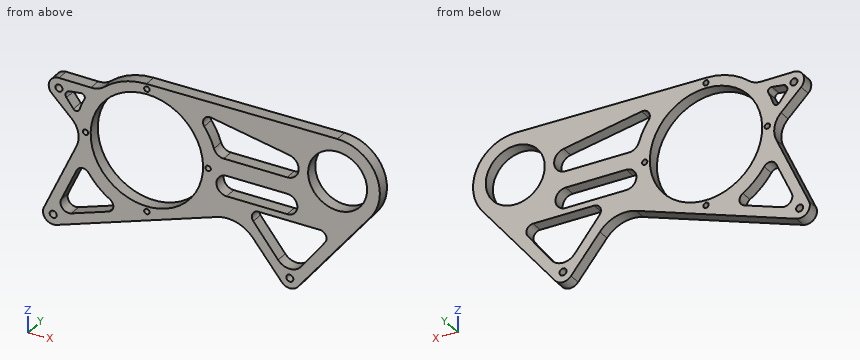
from build123d import *

# Parameters (mm, degrees)
SKETCH1_R             = 52.3875
SKETCH1_R_2           = 27.49999999
BOSS_EXTRUDE1_DEPTH   = 11.43
M6_CLEARANCE_HOLE1_D  = 6.6
F_5_0MM_DOWEL_HOLE1_D = 5
CIRPATTERN1_COUNT     = 4
CUT_EXTRUDE1_DEPTH    = 277.04812471
CUT_EXTRUDE2_DEPTH    = 277.04812471


with BuildPart() as part:
    # Sketch1 → Boss-Extrude1 (new body)
    with BuildSketch(Plane(origin=(0, 0, 0), x_dir=(1, 0, 0), z_dir=(0, 1, 0))):
        with BuildLine():
            Line((-207.352675902, -8.773903901), (-58.019530206, -60.290898352))
            ThreePointArc((-58.019530206, -60.290898352), (-39.599212065, -60.776397748), (-24.240097525, -50.595954211))
            Line((-24.240097525, -50.595954211), (2.624995443, -17.347825368))
            ThreePointArc((2.624995443, -17.347825368), (10.061549983, -13.809238065), (17.477288292, -17.391244328))
            Line((17.477288292, -17.391244328), (85.376811489, -102.435794114))
            ThreePointArc((85.376811489, -102.435794114), (90.030312626, -144.187156643), (54.354134393, -166.369168556))
            Line((54.354134393, -166.369168556), (-123.592369302, -165.212669907))
            ThreePointArc((-123.592369302, -165.212669907), (-144.74612022, -161.34018293), (-163.299086644, -150.465222234))
            ThreePointArc((-163.299086644, -150.465222234), (-168.867064733, -147.400846083), (-175.155117318, -146.477170878))
            Line((-175.155117318, -146.477170878), (-205.054266123, -146.707116576))
            ThreePointArc((-205.054266123, -146.707116576), (-213.929698734, -140.822073907), (-211.802405396, -130.387436669))
            Line((-211.802405396, -130.387436669), (-193.092894011, -112.008542149))
            ThreePointArc((-193.092894011, -112.008542149), (-187.088381157, -100.6982482), (-188.678110669, -87.991962988))
            Line((-188.678110669, -87.991962988), (-219.113977597, -21.755141651))
            ThreePointArc((-219.113977597, -21.755141651), (-217.51766362, -11.382814462), (-207.352675902, -8.773903901))
        make_face()
        with Locations(Location((-123.19, -103.30147742, 0), (0, 0, 270))):
            Circle(SKETCH1_R, mode=Mode.SUBTRACT)
        with Locations(Location((54.61, -127, 0), (0, 0, 270))):
            Circle(SKETCH1_R_2, mode=Mode.SUBTRACT)
    extrude(amount=BOSS_EXTRUDE1_DEPTH)

    # M6 Clearance Hole1 (through all)
    with Locations(Plane(origin=(0, 0, 0), x_dir=(-1, 0, 0), z_dir=(0, -1, 0))):
        with Locations((-10.033704867, -23.334197365), (210.458966133, -17.778157673), (205.127517975, -137.182398252)):
            Hole(M6_CLEARANCE_HOLE1_D / 2)

    # Ø5.0mm Dowel Hole1 (through all)
    with Locations(Plane(origin=(0, 0, 0), x_dir=(-1, 0, 0), z_dir=(0, -1, 0))):
        with Locations((123.19, -160.45147742)):
            f_5_0mm_dowel_hole1 = Hole(F_5_0MM_DOWEL_HOLE1_D / 2)

    # CirPattern1: Ø5.0mm Dowel Hole1 ×4 about axis
    cirpattern1_axis = Axis((-123.19, 0, 103.30147742), (0, 1, 0))
    for i in range(1, CIRPATTERN1_COUNT):
        add(f_5_0mm_dowel_hole1.rotate(cirpattern1_axis, i * 360 / CIRPATTERN1_COUNT), mode=Mode.SUBTRACT)

    # Sketch6 → Cut-Extrude1 (cut, through all)
    with BuildSketch(Plane.XZ):
        with BuildLine():
            Line((-23.944258321, 66.390441023), (-0.829614149, 37.099993387))
            ThreePointArc((-0.829614149, 37.099993387), (9.965816041, 31.919797806), (20.677978855, 37.270060145))
            Line((20.677978855, 37.270060145), (42.980839674, 66.469760223))
            ThreePointArc((42.980839674, 66.469760223), (43.626492897, 73.139052969), (37.934473227, 76.674197365))
            Line((37.934473227, 76.674197365), (-18.959475373, 76.674197365))
            ThreePointArc((-18.959475373, 76.674197365), (-24.673574285, 73.093957935), (-23.944258321, 66.390441023))
        make_face()
        with BuildLine():
            Line((-202.975515938, 34.064204485), (-188.656140545, 65.227105539))
            ThreePointArc((-188.656140545, 65.227105539), (-183.31891043, 68.976517371), (-177.425759363, 66.18100581))
            ThreePointArc((-177.425759363, 66.18100581), (-168.46871459, 55.664464381), (-157.511328264, 47.252450377))
            ThreePointArc((-157.511328264, 47.252450377), (-154.454895213, 41.026593051), (-158.781442678, 35.605885581))
            Line((-158.781442678, 35.605885581), (-193.515753631, 23.623232324))
            ThreePointArc((-193.515753631, 23.623232324), (-201.691580607, 25.721611775), (-202.975515938, 34.064204485))
        make_face()
        with BuildLine():
            Line((-195.382759208, 137.08408238), (-184.602414462, 138.548107412))
            ThreePointArc((-184.602414462, 138.548107412), (-181.561941078, 137.21737146), (-181.352428173, 133.905054912))
            ThreePointArc((-181.352428173, 133.905054912), (-183.92504724, 128.415239444), (-185.980839898, 122.711717787))
            ThreePointArc((-185.980839898, 122.711717787), (-188.468463156, 120.514659048), (-191.560851772, 121.719843357))
            Line((-191.560851772, 121.719843357), (-198.159072812, 130.369853834))
            ThreePointArc((-198.159072812, 130.369853834), (-198.701393345, 134.525214763), (-195.382759208, 137.08408238))
        make_face()
    extrude(amount=-CUT_EXTRUDE1_DEPTH, mode=Mode.SUBTRACT)

    # Sketch7 → Cut-Extrude2 (cut, through all)
    with BuildSketch(Plane.XZ):
        with BuildLine():
            Line((-48.815667356, 101.39647742), (7.572332644, 101.39647742))
            ThreePointArc((7.572332644, 101.39647742), (17.097332644, 91.87147742), (7.572332644, 82.34647742))
            Line((7.572332644, 82.34647742), (-48.815667356, 82.34647742))
            ThreePointArc((-48.815667356, 82.34647742), (-58.340667356, 91.87147742), (-48.815667356, 101.39647742))
        make_face()
        with BuildLine():
            Line((-63.185512617, 151.524232803), (9.527948512, 138.12987842))
            ThreePointArc((9.527948512, 138.12987842), (18.322585695, 126.531617281), (7.572332644, 116.718495252))
            Line((7.572332644, 116.718495252), (-51.525154545, 116.718495252))
            ThreePointArc((-51.525154545, 116.718495252), (-57.140513894, 118.54977285), (-60.59665397, 123.339442362))
            ThreePointArc((-60.59665397, 123.339442362), (-64.418746701, 132.718934684), (-69.636607751, 141.399786896))
            ThreePointArc((-69.636607751, 141.399786896), (-69.82125671, 148.634919104), (-63.185512617, 151.524232803))
        make_face()
    extrude(amount=-CUT_EXTRUDE2_DEPTH, mode=Mode.SUBTRACT)


solid = part.part
Geometry: final body of the model. Coordinates: model frame, mm. Round coordinates to 2 decimals unless told otherwise and drop trailing zeros. Loops run counter-clockwise (first coordinate to the right, second up) from the corner with the lowest first, then second, coordinate; pieces in that order, holes last.
Q1. Section D-D on y = 7.25. State how many separate pieces and enclosed holes the cut face has, plus the area to 3 significant figures.
Q2. Section A-A on z = 73.5. Return loops of the section in (x, y), plus the area to 3 significant figures.
Q3. Section C-C on z = 127. Return loops of the section in (x, y).
Q4. Section B-B on x = 30.5. Return loops of the section in (y, z), plus the area to 3 significant figures.
Q5. Material intervals for L1, parallel to X at y = 3.5, z = 74.5; L2, parallel to X at y = 5, z = 74; L3, parallel to X at y = 6, z = 68, sorted ascending.
Q6. Pin query (flat end, axial travel): P1, Ø3, axis at x = -123.19, z = 46.15, coming from the -Y side; P2, Ø5.5, axis at x = -26, y = 3.5, coming from the +Z side; P3, Ø2, axis at x = 53, y = 7, coming from the +Z side; P4, Ø6, axis at y = 3.5, z = 131, coming from the +X side. Return the tip coordinate at first contact, or that it passes through.
Evaluation:
1. separate pieces: 1
1. enclosed holes: 14
1. area: 16,400 mm2
2. outline: (-195.34, 0) - (-166.28, 0) - (-166.28, 11.43) - (-195.34, 11.43) - close; (-80.1, 0) - (-24.46, 0) - (-24.46, 11.43) - (-80.1, 11.43) - close; (43.43, 0) - (62.27, 0) - (62.27, 11.43) - (43.43, 11.43) - close
2. area: 1,180 mm2
3. outline: (-208.35, 0) - (-195.59, 0) - (-195.59, 11.43) - (-208.35, 11.43) - close; (-184.49, 0) - (-169.91, 0) - (-169.91, 11.43) - (-184.49, 11.43) - close; (-76.47, 0) - (-61.89, 0) - (-61.89, 11.43) - (-76.47, 11.43) - close; (18.36, 0) - (27.11, 0) - (27.11, 11.43) - (18.36, 11.43) - close; (82.11, 0) - (93.98, 0) - (93.98, 11.43) - (82.11, 11.43) - close
4. outline: (0, 33.7) - (11.43, 33.7) - (11.43, 50.13) - (0, 50.13) - close; (0, 76.67) - (11.43, 76.67) - (11.43, 113.77) - (0, 113.77) - close; (0, 140.23) - (11.43, 140.23) - (11.43, 166.21) - (0, 166.21) - close
4. area: 909 mm2
5. L1: x = -194.88 to -166.95, -79.43 to -23.74, 42.72 to 63.07
5. L2: x = -195.11 to -166.62, -79.76 to -24.14, 43.11 to 62.67
5. L3: x = -197.86 to -186.23, -179.31 to -161.9, -84.48 to -24.87, 43.84 to 57.88
6. P1: passes through
6. P2: stops at z = 165.86
6. P3: stops at z = 166.37
6. P4: stops at x = 93.97
